```python
from build123d import *

# Parameters (mm, degrees)
BOSS_EXTRU_1_DEPTH      = 10
ESQUISSE2_R             = 3.889151143
ENL_V_MAT_EXTRU_1_DEPTH = 89.737541713
ENL_V_MAT_EXTRU_2_DEPTH = 11


with BuildPart() as part:
    # Esquisse1 → Boss.-Extru.1 (new body)
    with BuildSketch(Plane.XY):
        Polygon((0, 0), (77.738226815, 0), (14.337114468, -88.737541713), (0, -88.737541713), align=None)
    extrude(amount=BOSS_EXTRU_1_DEPTH)

    # Esquisse2 → Enlèv. mat.-Extru.1 (cut, through all)
    with BuildSketch(Plane(origin=(0, 0, 0), x_dir=(1, 0, 0), z_dir=(0, 1, 0))):
        with Locations((7.959936212, -5.179369155)):
            Circle(ESQUISSE2_R)
    extrude(amount=-ENL_V_MAT_EXTRU_1_DEPTH, mode=Mode.SUBTRACT)

    # Esquisse4 → Enlèv. mat.-Extru.2 (cut, through all)
    with BuildSketch(Plane.XY.offset(10)):
        Polygon((13.992554962, -9.272968918), (13.992554962, -71.289178), (61.99380154, -9.272968918), align=None)
    extrude(amount=-ENL_V_MAT_EXTRU_2_DEPTH, mode=Mode.SUBTRACT)


solid = part.part
```
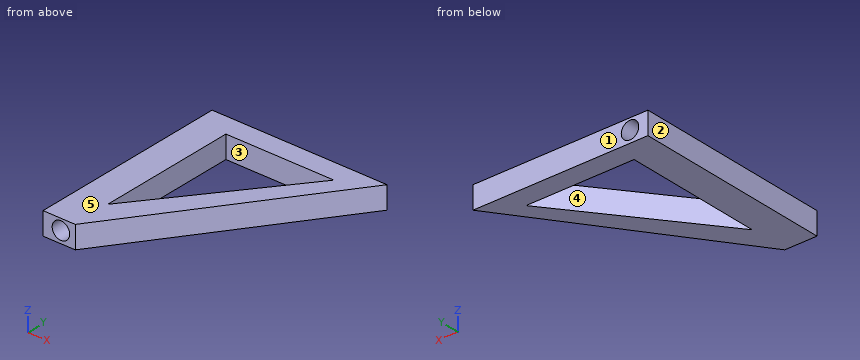
Geometry: final body of the model. Coordinates: model frame, mm. Face numbers are marked on the shaded views. A direction names the side the tool comes from. Round coordinates to 2 decimals unless told otherwise and drop trailing zeros. Order: outer loops, then holes, each group sorted by start corner. A loop starts at its lowest first (then second) coordinate and runs counter-clockwise, first axis right, second up. Notation, with made-up numbers: (20, 64.25) -> (36, 64.25) arc R23 cw to (36, 85.25) -> close; hole circle Ø4 at (-30, 74.5). An arc over 180 degrees is marked (long way). Use one line per item in the form item = value. Start each with the question number.
1. Reachability of the marked faces 4 and 5 from +Z, -Z, +X, -X, +Y, -Y: full face, straight path, thin tool, end or side. Return the list, or none.
2. Cut plane D-D (y = -65). Return the cut outline in (x, z), then the cut area to 3 significant figures.
3. Line query: probe 1 along X at (y, z) = (-48.5, 5.5); probe 2 along X at (y, z) = (-17, 8); probe 3 along Y at (x, z) = (15.5, 5.75). Output: solid intervals per line, ascending.
4. Cut plane A-A (y = -16). Return the cut outline in (x, z), then the cut area to 3 significant figures.
5. Cut plane C-C (x = 39). Return the cut outline in (y, z).
6. Draft query along Y for the marked faces 1, 2 and 3. Return one class per face: pulls with the +Y half, pulls with the -Y half, needs draft (parallel to the pull), parting line crosses it, or undercut.
7. Cut plane B-B (z = 3.5). Return the cut outline in (x, y).
8. Pin query (flat end, axial travel): pin 1 Ø4 at (y, z) = (-65, 2.5) entering from -X; pin 2 Ø2 at (y, z) = (-13.5, 5) entering from +X. Return the tip coordinate at first contact, or that it passes through.
Solution:
q1.face_4 = +Z, -Z
q1.face_5 = +Z, +X, -X, +Y, -Y
q2.outline = (0, 0) -> (13.99, 0) -> (13.99, 10) -> (0, 10) -> close; (18.86, 0) -> (31.3, 0) -> (31.3, 10) -> (18.86, 10) -> close; hole circle Ø7.78 at (7.96, 5.18)
q2.area = 217 mm^2
q3.probe_1 = 0 to 4.08, 11.84 to 13.99, 31.63 to 43.09
q3.probe_2 = 0 to 5.28, 10.64 to 13.99, 56.01 to 65.59
q3.probe_3 = -87.11 to -69.34, -9.27 to 0
q4.outline = (0, 0) -> (13.99, 0) -> (13.99, 10) -> (0, 10) -> close; (56.79, 0) -> (66.31, 0) -> (66.31, 10) -> (56.79, 10) -> close; hole circle Ø7.78 at (7.96, 5.18)
q4.area = 188 mm^2
q5.outline = (-54.22, 0) -> (-38.98, 0) -> (-38.98, 10) -> (-54.22, 10) -> close; (-9.27, 0) -> (0, 0) -> (0, 10) -> (-9.27, 10) -> close
q6.face_1 = pulls with the +Y half
q6.face_2 = needs draft
q6.face_3 = undercut
q7.outline = (0, -88.74) -> (4.45, -88.74) -> (4.45, 0) -> (0, 0) -> close; (11.47, -88.74) -> (14.34, -88.74) -> (77.74, 0) -> (11.47, 0) -> close; hole (13.99, -71.29) -> (61.99, -9.27) -> (13.99, -9.27) -> close
q8.pin_1 = 0
q8.pin_2 = 68.81
